Source: three-view drawing plus pictorial views. Frame: mm from the lowest corner of the part. A direction names the side the tool comes from. Round coordinates to 2 decimals unless told otherwise and drop trailing zeros. Write each loop counter-clockwise with the first axis right and the second up, starting at its lowest first coordinate (ties: lowest second). Pieces come first, ordered by that corner, then holes. Notation, with made-up numbers: M -33,-11.5 L 16,-11.5 A14 ccw 16,-1.5 Z; hole C 57.25,88.5 d2. An arc over 180 degrees is marked long. Answer in a Markdown table with one row per item.
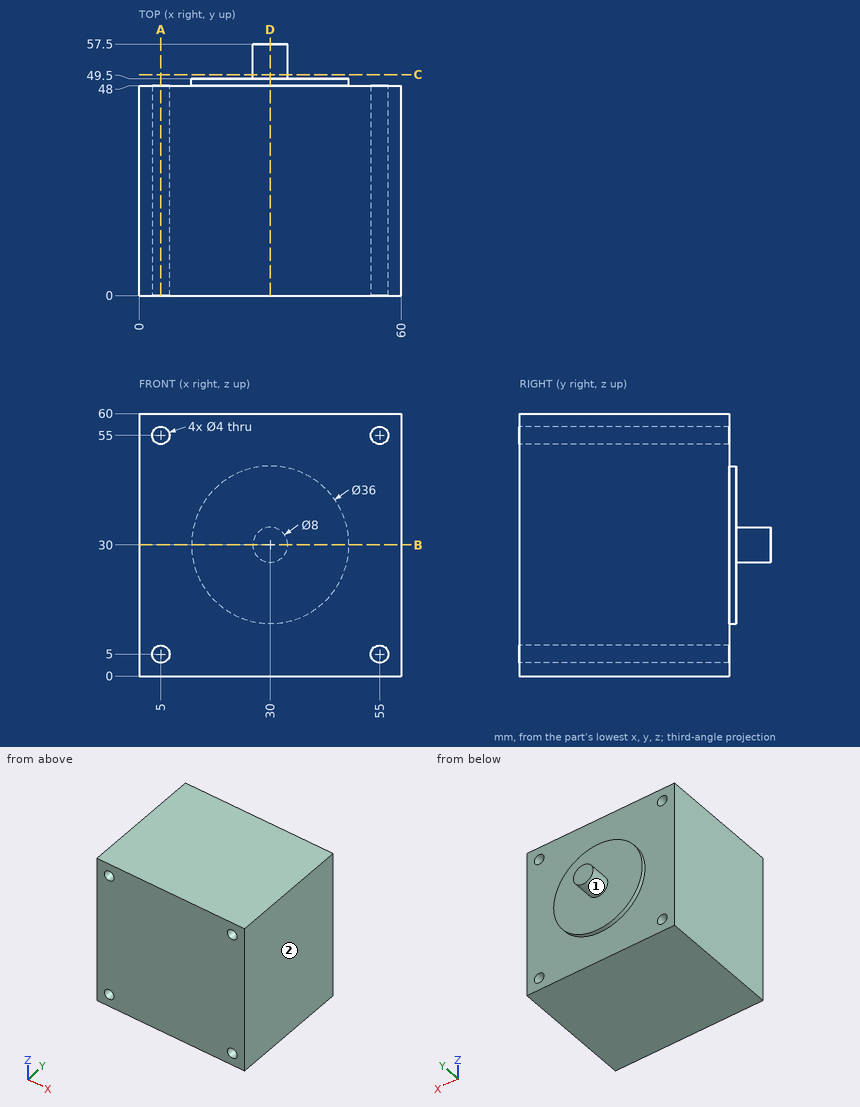
Q1. Access query for the marked faces 1 and 2. Directions: +Z, -Z, +X, -X, +Y, -Y. A direction counts if a zero-diameter tool reaches every point of the face in a straight line with its end or side. Return the directions, or none.
Solutions:
| item | result |
|---|---|
| face 1 | +Y |
| face 2 | +Z, -Z, +X, +Y, -Y |
Q2. Section A-A (x = 5). Return loops of the section in (y, z), and give its area (3 significant figures).
Solutions:
| item | result |
|---|---|
| outline | M 0,0 L 48,0 L 48,3 L 0,3 Z; M 0,7 L 48,7 L 48,53 L 0,53 Z; M 0,57 L 48,57 L 48,60 L 0,60 Z |
| area | 2,500 mm2 |
Q3. Contact query for flat-ended pins moving along their axis: pin 1 Ø8 at (y, z) = (38.5, 42) entering from -X; pin 2 Ø2 at (x, z) = (19, 7.5) entering from +Y. Output: stop coordinate, or through.
Solutions:
| item | result |
|---|---|
| pin 1 | stops at x = 0 |
| pin 2 | stops at y = 48 |
Q4. Section B-B (z = 30). Return loops of the section in (x, y).
Solutions:
| item | result |
|---|---|
| outline | M 0,0 L 60,0 L 60,48 L 48,48 L 48,49.5 L 34,49.5 L 34,57.5 L 26,57.5 L 26,49.5 L 12,49.5 L 12,48 L 0,48 Z |
Q5. Section D-D (x = 30). Return loops of the section in (y, z).
Solutions:
| item | result |
|---|---|
| outline | M 0,0 L 48,0 L 48,12 L 49.5,12 L 49.5,26 L 57.5,26 L 57.5,34 L 49.5,34 L 49.5,48 L 48,48 L 48,60 L 0,60 Z |
Q6. Section C-C (y = 50.5). Return loops of the section in (x, z).
Solutions:
| item | result |
|---|---|
| outline | C 30,30 d8 |
Q7. Material intervals for probe 1 along X at (y, z) = (31, 5); probe 2 along X at (y, z) = (41, 54), sorted ascending.
Solutions:
| item | result |
|---|---|
| probe 1 | x = 0 to 3, 7 to 53, 57 to 60 |
| probe 2 | x = 0 to 3.27, 6.73 to 53.27, 56.73 to 60 |
